Source: CAD feature listing. Evaluate the final solid. Frame: model axes, mm. Face numbers are marked on the shaded views. A direction names the side the tool comes from. Round coordinates to 2 decimals unless told otherwise and drop trailing zeros. Order: outer loops, then holes, each group sorted by start corner. A loop starts at its lowest first (then second) coordinate and runs counter-clockwise, first axis right, second up. Notation, with made-up numbers: M 16.5,-40 L 45.5,-40 A36 ccw 45.5,-3 Z; hole C -13.5,27.25 d10. An arc over 180 degrees is marked long. Answer in a Markdown table with one row per item. Add a question column.
Autodesk Inventor part; units mm, degrees
ref_plane "YZ Plane" through (0, 0, 0) normal (1, 0, 0) x (0, 1, 0)
ref_plane "XZ Plane" through (0, 0, 0) normal (0, 1, 0) x (-1, 0, 0)
ref_plane "XY Plane" through (0, 0, 0) normal (0, 0, 1) x (1, 0, 0)
sketch "Sketch1" plane through (0, 0, 0) normal (0, 0, 1) x (1, 0, 0)
  line L0 (-5.375, -2) -> (5.375, -2)
  line L1 (5.375, -2) -> (5.375, 2)
  line L2 (5.375, 2) -> (-5.375, 2)
  line L3 (-5.375, 2) -> (-5.375, -2)
  line L4 (-5.375, -2) -> (5.375, 2) construction
  line L5 (5.375, -2) -> (-5.375, 2) construction
  point P0 (0, 0)
  dimension "d0" = 10.75
  dimension "d1" = 4
extrude "Extrusion1" add sketch "Sketch1" along normal blind 7.7
sketch "Sketch2" plane through (0, 0, 0) normal (0, 0, -1) x (-1, 0, 0)
  line L0 (5.375, -2) -> (-5.375, -2)
  line L1 (5.375, 2) -> (5.375, -2)
  line L2 (-5.375, 2) -> (5.375, 2)
  line L3 (-5.375, -2) -> (-5.375, 2)
  line L4 (6.25, 2) -> (-6.25, 2)
  line L5 (-6.25, 2) -> (-6.25, -3)
  line L6 (-6.25, -3) -> (6.25, -3)
  line L7 (6.25, -3) -> (6.25, 2)
  point P0 (0, 0)
  dimension "d4" = 0.875
  dimension "d6" = 0.875
  dimension "d7" = 1
extrude "Extrusion2" add sketch "Sketch2" against normal blind 0.9 contours L1 L4 L7 L6 L5 L3 L0
sketch "Sketch3" plane through (0, 0, 7.7) normal (0, 0, 1) x (1, 0, 0)
  line L0 (-5.375, 2) -> (-5.375, -2)
  line L1 (5.375, -2) -> (-5.375, -2)
  line L2 (-5.375, -2) -> (-5.375, -0.25)
  line L3 (-5.375, -0.25) -> (5.375, -0.25)
  line L4 (5.375, -0.25) -> (5.375, -2)
  point P0 (0, 0)
  dimension "d10" = 1.75
extrude "Extrusion3" add sketch "Sketch3" along normal blind 0.3
sketch "Sketch4" plane through (0, 0, 8) normal (0, 0, 1) x (1, 0, 0)
  line L0 (-5.375, -2) -> (5.375, -2)
  line L1 (-4.375, -2) -> (-4.25, -1)
  line L2 (-4.25, -1) -> (-3, -1)
  line L3 (-3, -1) -> (-2.875, -2)
  point P0 (0, 0)
  dimension "d13" = 1
  dimension "d14" = 1
  dimension "d15" = 1.5
  dimension "d16" = 1.25
extrude "Extrusion4" cut sketch "Sketch4" against normal blind 3.25
pattern_linear "Rectangular Pattern1" count 4 spacing 2.4167 along (1, 0, 0) of "Extrusion4"
sketch "Sketch5" plane through (0, 0, 7.7) normal (0, 0, 1) x (1, 0, 0)
  line L0 (-5.375, 2) -> (-5.375, -0.25)
  line L1 (-3.075, 0.325) -> (-4.175, 0.325)
  line L2 (-4.175, 0.325) -> (-4.175, 1.425)
  line L3 (-4.175, 1.425) -> (-3.075, 1.425)
  line L4 (-3.075, 1.425) -> (-3.075, 0.325)
  line L5 (-3.075, 0.325) -> (-4.175, 1.425) construction
  line L6 (-4.175, 0.325) -> (-3.075, 1.425) construction
  line L7 (-4.25, -1) -> (-3, -1)
  point P0 (0, 0)
  point P1 (-3.625, 0.875)
  point P2 (-3.625, 0.875)
  point P3 (-5.375, 0.875)
  point P4 (-3.625, -1)
  point P5 (-3.625, 0.875)
  dimension "d23" = 1.1
extrude "Extrusion5" cut sketch "Sketch5" against normal through all
pattern_linear "Rectangular Pattern2" count 4 spacing 2.4167 along (1, 0, 0) of "Extrusion5"
sketch "Sketch6" plane through (0, 0, 0) normal (0, 0, -1) x (-1, 0, 0)
  line L0 (-2.525, -1.175) -> (-2.525, 1.425)
  line L1 (-2.525, 1.425) -> (-4.725, 1.425)
  line L2 (-4.725, 1.425) -> (-4.725, -1.175)
  line L3 (-4.185, -1.175) -> (-4.185, -1.675)
  line L4 (-4.185, -1.675) -> (-3.065, -1.675)
  line L5 (-3.065, -1.675) -> (-3.065, -1.175)
  line L6 (-4.725, -1.175) -> (-4.185, -1.175)
  line L7 (-3.065, -1.175) -> (-2.525, -1.175)
  line L8 (-4.375, -2) -> (-2.875, -2)
  line L9 (-4.25, -1) -> (-4.375, -2)
  line L10 (-3, -1) -> (-4.25, -1)
  line L11 (-2.875, -2) -> (-3, -1)
  line L12 (-1.9583, -2) -> (-0.4583, -2)
  line L13 (-1.8333, -1) -> (-1.9583, -2)
  line L14 (-0.5833, -1) -> (-1.8333, -1)
  line L15 (-0.4583, -2) -> (-0.5833, -1)
  point P0 (-3.625, 1.425)
  point P1 (-3.625, -1.675)
  point P2 (-3.625, -1)
  point P3 (-1.2083, -1)
  point P4 (-4.175, 1.425)
  dimension "d31" = 2.2
  dimension "d34" = 1.12
  dimension "d37" = 0.5
  dimension "d38" = 2.6
  dimension "d56" = 2.4167
sketch "Sketch7" plane through (-5.375, 2, 7.7) normal (0, 1, 0) x (1, 0, 0)
  line L0 (-0.875, 7.7) -> (11.625, 7.7)
  line L1 (10.75, 0) -> (0, 0)
  line L2 (10.75, 6.8) -> (10.75, 0)
  line L3 (8.335, 6.8) -> (9.185, 6.8)
  line L4 (8.335, 3.75) -> (9.985, 3.75)
  line L5 (9.985, 3.75) -> (9.5174, 1.55)
  line L6 (9.5174, 1.55) -> (8.335, 1.55)
  line L7 (8.335, 6.8) -> (8.335, 1.55)
  line L8 (9.185, 6.8) -> (9.585, 3.75)
  line L9 (5.375, 7.7) -> (5.375, 0)
  line L10 (9.185, 6.8) -> (9.067, 7.7)
  line L11 (5.375, 7.7) -> (9.067, 7.7)
  line L12 (8.335, 6.8) -> (5.375, 6.8)
  point P0 (5.375, 7.7)
  dimension "d41" = 0.85
  dimension "d45" = 1.25
  dimension "d46" = 6.15
  dimension "d48" = 2.2
  dimension "d49" = 12
  dimension "d50" = 0.4
  dimension "d52" = 5.92
  dimension "d53" = 0.9
extrude "Extrusion6" add sketch "Sketch7" along normal blind 0.85
mirror "Mirror1" about plane through (0, 0, 0) normal (1, 0, 0) of "Extrusion6"
extrude "Extrusion7" cut sketch "Sketch6" against normal blind 4.5 contours L7 L11 L10 L9 L6 L2 L1 L0 | L7 L5 L4 L3 L6 L9 L10 L11
pattern_linear "Rectangular Pattern3" count 4 spacing 2.4167 along (-1, 0, 0) of "Extrusion7"
sketch "Sketch8" plane through (0, 0, 0.9) normal (0, 0, 1) x (1, 0, 0)
  line L0 (6.25, -3) -> (6.25, 2)
  line L1 (6.25, -0.85) -> (6.25, -0.15)
  line L2 (6.25, -0.85) -> (5.75, -0.5)
  line L3 (5.75, -0.5) -> (6.25, -0.15)
  point P0 (0, 0)
  point P1 (6.25, -0.5)
  point P2 (6.25, -0.5)
  dimension "d63" = 0.7
  dimension "d64" = 0.5
extrude "Extrusion8" cut sketch "Sketch8" against normal through all
equation "\"d29\" = d21"
equation "\"d61\" = d21"
properties part number "3S Female JST XH 4 Pin" material "PBT Plastic"
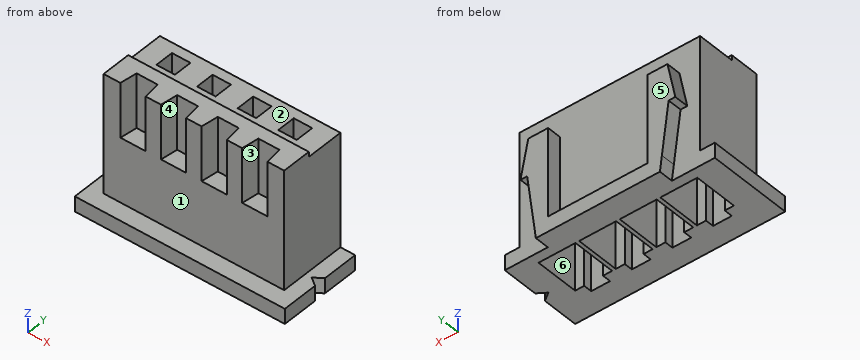
(1) Draft query along Y for the marked faces 4, 5 and 6. Return one class per face: +Y half, -Y half, draft (parallel to the pull), parting line (faces both ways), or undercut.
(2) Line query: line 1 (X direction, y = 0.5, z = 1.5) (3 decimals); line 2 (X direction, y = -1.5, z = 2.5) (3 decimals); line 3 (Y direction, x = 1.25, z = 3) (3 decimals). Output: solid intervals per line, ascending. Write a range as from..to.
(3) Cut plane B-B (y = 2.35). Return loops of the section in (x, z), and give its area (3 significant figures).
(4) Cut plane A-A (x = 1). Return loops of the section in (y, z) (3 decimals).
(5) Pin query (flat end, axial travel): pin 1 (1.8 mm diameter, centred on x = -3, z = 3.5, fed in from -Y); pin 2 (1.1 mm diameter, centred on x = 1.5, y = -0.5, fed in from -Z); pin 3 (2 mm diameter, centred on y = 0.5, z = 2, fed in from +X) (3 decimals). Return the tip coordinate at first contact, or that it passes through.
(6) Cut plane C-C (z = 6.75). Count the separate pieces of the cut face and the enclosed holes in it, and give its area (3 significant figures).
(7) Access query for the marked faces 1, 2 and 3. Directions: +Z, -Z, +X, -X, +Y, -Y. A direction counts if a zero-diameter tool reaches every point of the face in a straight line with its end or side. Return the directions, or none.
Answer list:
| question | item | result |
|---|---|---|
| 1 | face 4 | -Y half |
| 1 | face 5 | +Y half |
| 1 | face 6 | undercut |
| 2 | line 1 | -5.375..-4.725, -2.525..-2.308, -0.108..0.108, 2.308..2.525, 4.725..5.375 |
| 2 | line 2 | -5.375..-4.185, -3.065..-1.768, -0.648..0.648, 1.768..3.065, 4.185..5.375 |
| 2 | line 3 | -2..-1.675, 1.425..2 |
| 3 | outline | M -4.61,3.95 L -4.21,3.95 L -3.81,0.9 L -3.69,0 L 3.69,0 L 3.81,0.9 L 4.21,3.95 L 4.61,3.95 L 4.14,6.15 L 2.96,6.15 L 2.96,0.9 L -2.96,0.9 L -2.96,6.15 L -4.14,6.15 Z |
| 3 | area | 19.4 mm² |
| 4 | outline | M -3,0 L -1.675,0 L -1.675,4.5 L 0.325,4.5 L 0.325,7.7 L -0.25,7.7 L -0.25,8 L -1,8 L -1,4.75 L -2,4.75 L -2,0.9 L -3,0.9 Z; M 1.425,0 L 2.85,0 L 2.85,0.9 L 2,0.9 L 2,7.7 L 1.425,7.7 Z |
| 5 | pin 1 | y = -2 |
| 5 | pin 2 | z = 4.5 |
| 5 | pin 3 | x = 5.375 |
| 6 | separate pieces | 1 |
| 6 | enclosed holes | 4 |
| 6 | area | 32.7 mm² |
| 7 | face 1 | +Z, +X, -X, -Y |
| 7 | face 2 | +Z, +X, -X, +Y |
| 7 | face 3 | +Z, -Y |
